```python
from build123d import *

# Parameters (mm, degrees)
SKETCH1_W           = 19.05
SKETCH1_H           = 139.7
BOSS_EXTRUDE1_DEPTH = 1.016
SKETCH2_R           = 3.175
CUT_EXTRUDE1_DEPTH  = 141.028025341
BOSS_EXTRUDE2_START = -19.05
BOSS_EXTRUDE2_DEPTH = 19.05
CUT_EXTRUDE2_DEPTH  = 142.362614158
FILLET1_R           = 10.16


# Read off the part's stored shape, not the designer's step: Boss-Extrude2
with BuildPart() as part:
    # Sketch1 → Boss-Extrude1 (new body)
    with BuildSketch(Plane.XY):
        with Locations((0, 69.85)):
            Rectangle(SKETCH1_W, SKETCH1_H)
    extrude(amount=BOSS_EXTRUDE1_DEPTH)

    # Sketch2 → Cut-Extrude1 (cut, through all)
    with BuildSketch(Plane.XY.offset(1.016)):
        with Locations((0, 107.95)):
            Circle(SKETCH2_R)
    extrude(amount=-CUT_EXTRUDE1_DEPTH, mode=Mode.SUBTRACT)

    # Boss-Extrude2 outline → Boss-Extrude2 (add)
    with BuildSketch(Plane(origin=(9.525, 0, 0), x_dir=(0, 0, -1), z_dir=(1, 0, 0)).offset(BOSS_EXTRUDE2_START)):
        with BuildLine():
            add(Edge.make_bspline(
                [(-1e-08, 89.021856582), (0.353951992, 87.40678329), (1.153670007, 84.14800116), (2.913866895, 77.737270865), (5.184849484, 69.73490743), (7.461415384, 59.944664253), (9.047721746, 49.78686922), (9.924339704, 39.212202023), (10.183044993, 30.10799928), (10.225102879, 22.747853486), (10.207581307, 17.22630398), (10.179157942, 12.664005658), (10.163337481, 9.05650551), (10.16, 7.285124222), (10.16, 6.395385599)],
                knots=[0.00134616, 0.00134616, 0.00134616, 0.00134616, 0.0625, 0.125, 0.25, 0.375, 0.5, 0.625, 0.75, 0.8125, 0.875, 0.9375, 0.96875, 1, 1, 1, 1], degree=3))
            Line((-1e-08, 89.021856582), (0, 84.644701296))
            add(Edge.make_bspline(
                [(0, 84.644701296), (3.804384443, 69.740616889), (9.143429465, 56.08795928), (9.602178505, 40.318745924), (9.144, 22.473473321), (9.144, 6.395385599)],
                knots=[0.053605471, 0.053605471, 0.053605471, 0.053605471, 0.053605471, 0.053605471, 1, 1, 1, 1, 1, 1], degree=5))
            Line((9.144, 6.395385599), (9.144, 0))
            Line((9.144, 0), (10.16, 0))
            Line((10.16, 0), (10.16, 6.395385599))
        make_face()
    extrude(amount=BOSS_EXTRUDE2_DEPTH)

    # Sketch4 → Cut-Extrude2 (cut, through all)
    with BuildSketch(Plane(origin=(9.525, 0, 0), x_dir=(0, 0, -1), z_dir=(1, 0, 0))):
        with BuildLine():
            Line((-1.016, 90.953756608), (-1.016, 0))
            Line((-1.016, 0), (0, 0))
            Line((0, 0), (0, 84.644701296))
            add(Edge.make_bspline(
                [(0, 84.644701296), (-1.016, 87.704234075), (-1.016, 90.953756608)],
                knots=[0, 0, 0, 1, 1, 1], degree=2))
        make_face()
    extrude(amount=-CUT_EXTRUDE2_DEPTH, mode=Mode.SUBTRACT)

    # Fillet1
    fillet1_edges = [part.edges().sort_by_distance(p)[0] for p in [
        (0, 89.021856582, 1e-08),
    ]]
    fillet(fillet1_edges, radius=FILLET1_R)


solid = part.part
```
Input: part model. Units: mm. Frame: model coordinates. A direction names the side the tool comes from. Round coordinates to 2 decimals unless told otherwise and drop trailing zeros. Loops run counter-clockwise (first coordinate to the right, second up) from the corner with the lowest first, then second, coordinate; pieces in that order, holes last. Notation, with made-up numbers: M -19,-12.5 L -11,-12.5 A32 cw -11,22.5 Z; hole C -28.5,-14.5 d6. An arc over 180 degrees is marked long. Answer in a Markdown table with one row per item. Add a question column.
1. Contact query for flat-ended pins moving along their axis: pin 1 (1.9 mm diameter, centred on x = -0.5, y = 4, fed in from +Z); pin 2 (1 mm diameter, centred on x = -6.5, y = 86, fed in from -Z); pin 3 (3 mm diameter, centred on y = 57, z = -4, fed in from -X); pin 4 (2 mm diameter, centred on x = -5.5, y = 108, fed in from -Z). Output: stop coordinate, or through.
2. Section A-A (y = 107.95). Output: boundary loops of the cut face in (x, z) (3 decimals).
3. Ray query, probe 1 along Z at (x, y) = (2.5, 9); probe 2 along Z at (x, y) = (-4.5, 123.5). Return the intervals inside material, ascending.
4. Mould query, pull axis Y, two halves, no side actions, for faces 3 (the face through (0, 116, 1.016)), 4 (the face through (-0.69, 104.85, 0.52)). Classes: released by +Y, released by -Y, zero draft, split by the parting line, or undercut.
5. Set-up query: faces 1 (the face through (0, 3, -9.144)), 2 (the face through (0, 115, 0)). Return all of +Z, -Z, +X, -X, +Y, -Y with unobstructed straight access to the full face (end or side cutting, diameter ignored); none if empty.
Values follow:
| question | item | result |
|---|---|---|
| 1 | pin 1 | z = -9.14 |
| 1 | pin 2 | z = -0.83 |
| 1 | pin 3 | through |
| 1 | pin 4 | z = 0 |
| 2 | outline | M -9.525,0 L -3.175,0 L -3.175,1.016 L -9.525,1.016 Z; M 3.175,0 L 9.525,0 L 9.525,1.016 L 3.175,1.016 Z |
| 3 | probe 1 | -10.16 to -9.15 |
| 3 | probe 2 | 0 to 1.02 |
| 4 | face 3 | zero draft |
| 4 | face 4 | undercut |
| 5 | face 1 | +Z, +X, -X, -Y |
| 5 | face 2 | -Z, +X, -X, +Y |
